```python
from build123d import *

# Parameters (mm, degrees)
SKETCH_2_R      = 15
EXTRUDE_2_DEPTH = 41
SKETCH_5_R      = 25
EXTRUDE_4_DEPTH = 9
EXTRUDE_START   = -9
SKETCH_6_R      = 25
EXTRUDE_5_DEPTH = 60


with BuildPart() as part:
    # Эскиз2 → Бобышка-Вытянуть2 (new body)
    with BuildSketch(Plane(origin=(0, 0, 0), x_dir=(0, 0, -1), z_dir=(1, 0, 0))):
        Circle(SKETCH_2_R)
        with BuildLine():
            Line((2.5, 10.8), (2.5, 7.599342077))
            ThreePointArc((2.5, 7.599342077), (6.480740698, 4.69041576), (8, 0))
            ThreePointArc((8, 0), (-4.69041576, -6.480740698), (-2.5, 7.599342077))
            Line((-2.5, 7.599342077), (-2.5, 10.8))
            Line((-2.5, 10.8), (0, 10.8))
            Line((0, 10.8), (2.5, 10.8))
        make_face(mode=Mode.SUBTRACT)
    extrude(amount=EXTRUDE_2_DEPTH)

    # Эскиз5 → Бобышка-Вытянуть4 (add)
    with BuildSketch(Plane(origin=(0, 0, 0), x_dir=(0, 0, -1), z_dir=(1, 0, 0))):
        Circle(SKETCH_5_R)
    extrude(amount=-EXTRUDE_4_DEPTH)

    # Эскиз6 → Бобышка-Вытянуть5 (add)
    with BuildSketch(Plane(origin=(0, 0, 0), x_dir=(0, 0, -1), z_dir=(1, 0, 0)).offset(EXTRUDE_START)):
        Circle(SKETCH_6_R)
        with BuildLine():
            ThreePointArc((14, 0), (-8.366600265, -11.22497216), (-4, 13.416407865))
            Line((-4, 13.416407865), (-4, 17.3))
            Line((-4, 17.3), (0, 17.3))
            Line((0, 17.3), (4, 17.3))
            Line((4, 17.3), (4, 13.416407865))
            ThreePointArc((4, 13.416407865), (11.22497216, 8.366600265), (14, 0))
        make_face(mode=Mode.SUBTRACT)
    extrude(amount=-EXTRUDE_5_DEPTH)

    # Эскиз7 → Повернуть1 (revolve)
    with BuildSketch(Plane(origin=(0, 0, 0), x_dir=(1, 0, 0), z_dir=(0, 1, 0)), mode=Mode.PRIVATE) as revolve_1_sk:
        Polygon((0, 25), (0, 15), (41, 15), align=None)
    revolve(revolve_1_sk.sketch.rotate(Axis((-60.197075593, 0, 0), (1, 0, 0)), 180), axis=Axis((-60.197075593, 0, 0), (1, 0, 0)))


solid = part.part
```
Geometry check sheet. Reference: the model listing, model coordinates, mm. A direction names the side the tool comes from. Give positions to 0.01 mm unless a question says otherwise; leave off trailing zeros. Order: outer loops, then holes, each group sorted by start corner. A loop starts at its lowest first (then second) coordinate and runs counter-clockwise, first axis right, second up. Notation, with made-up numbers: (38.25, 35) - (42.25, 35) arc R22 ccw to (42.25, 67) - close; hole circle Ø5 at (30, 56). An arc over 180 degrees is marked (long way). Write item = value, one per line. Start each with the question number.
1) Draft check along Y on faces 4 (the conical face through (24.769, -5.695, 18.083)), 5 (the flat face through (-69, -11, -11)), 6 (the flat face through (-39, 15, 4)). Enter one of: released by +Y, released by -Y, zero draft, split by the parting line, or undercut.
2) Section check A-A (x = -32). Enter the section's corners in (y, z).
3) Section check C-C (x = 22). Enter the section's corners in (y, z), then the cut area to 3 significant figures.
4) Section check B-B (z = 0). Enter the section's corners in (x, y), then the cut area to 3 significant figures.
5) Access from +Z, -Z, +X, -X, +Y, -Y to the whole of each face (thin tool, end or side, straight path). Record for faces 1 (the flat face through (0, 2, 0)), 2 (the flat face through (41, -6, -6)), 3 (the flat face through (-39, 17.3, 0)).
6) Scan lines: L1, parallel to Z at x = -31, y = 20; L2, parallel to X at y = 5, z = 3; L3, parallel to X at y = -11, z = -0.5. Record each from-to range of solid material in increasing order.
7) Gauge pin test, flat ends, axial feed: pin 1 Ø4 at (x, z) = (24, -1) entering from -Y; pin 2 Ø3 at (x, z) = (-55, -12) entering from +Y; pin 3 Ø14 at (y, z) = (-3.5, 2.5) entering from -X. Record the tip position at first contact, or that the pin passes through.
Geometry check:
q1.face_4 = split by the parting line
q1.face_5 = zero draft
q1.face_6 = undercut
q2.outline = circle Ø50 at (0, 0); hole (13.42, -4) - (17.3, -4) - (17.3, 4) - (13.42, 4) arc R14 ccw (long way) to start
q3.outline = circle Ø39.27 at (0, 0); hole (7.6, -2.5) - (10.8, -2.5) - (10.8, 2.5) - (7.6, 2.5) arc R8 ccw (long way) to start
q3.area = 995 mm2
q4.outline = (-69, -25) - (0, -25) - (41, -15) - (41, -8) - (0, -8) - (0, 10.8) - (41, 10.8) - (41, 15) - (0, 25) - (-69, 25) - (-69, 17.3) - (-9, 17.3) - (-9, -14) - (-69, -14) - close
q4.area = 2,440 mm2
q5.face_1 = +X
q5.face_2 = +Z, -Z, +X, +Y, -Y
q5.face_3 = -X
q6.L1 = -15 to 15
q6.L2 = -9 to 0
q6.L3 = -9 to 41
q7.pin_1 = -19.62
q7.pin_2 = 22.69
q7.pin_3 = -9
